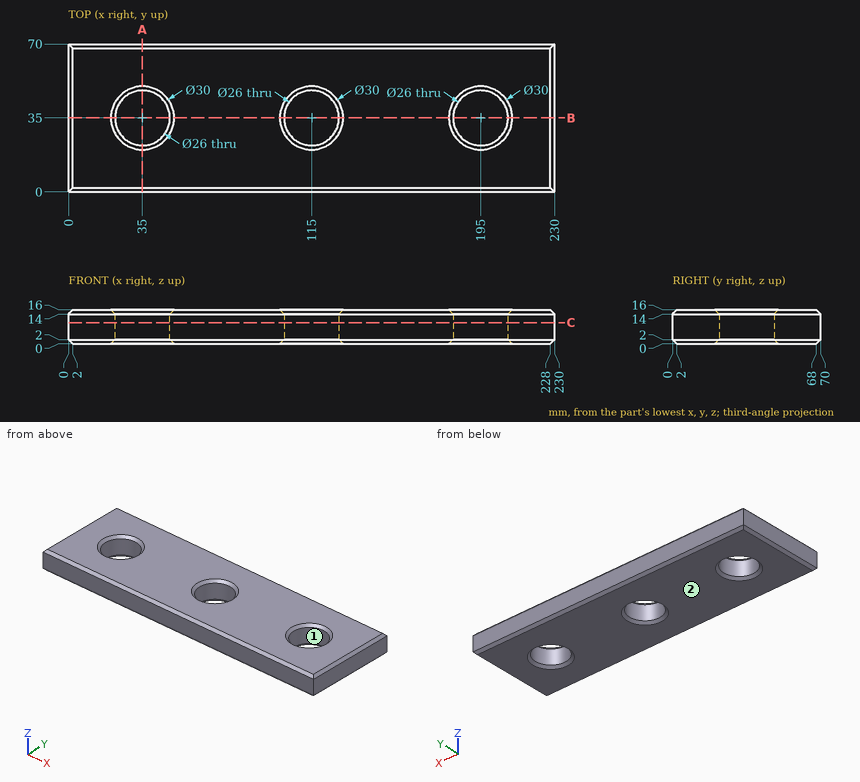
Here's the drawing with two shaded views (mm, measured from the low corner). I have some questions. Round coordinates to 2 decimals unless told otherwise and drop trailing zeros. Order: outer loops, then holes, each group sorted by start corner. A loop starts at its lowest first (then second) coordinate and runs counter-clockwise, first axis right, second up. Notation, with made-up numbers: (82.5, 10) -> (125.5, 10) arc R13 cw to (125.5, 29) -> close; hole circle Ø6 at (-13, 35.5). An arc over 180 degrees is marked (long way). Use a Markdown table: item, result. Add a question column.
(1) Suppose I cut it at C-C, the plane z = 10. Please give me the cut outline in (x, y), and give its area (3 significant figures).
(2) For pin 1 Ø12 at (x, y) = (34, 42.5) entering from -Z; pin 2 Ø10 at (x, y) = (197, 26.5) entering from -Z, each with a flat end and sliding along its axis, tell me the tip position at first contact or that it passes through.
(3) If we mould it in two halves opening along X, with no side actions, what happens to the marked faces 1 and 2? For each: released by +X, released by -X, zero draft, split by the parting line, or undercut.
(4) Suppose I cut it at B-B, the plane y = 35. Count the separate pieces of the cut face and the enclosed holes in it, and give its area (3 significant figures).
(5) I need wall thicknesses on line 1 along X through (y, z) = (34, 6); line 2 along Y through (x, z) = (195, 9); line 3 along X through (y, z) = (41, 6). Which ranges of each line are inside material? Lowest first, please.
(6) Suppose I cut it at A-A, the plane x = 35. Please give me the cut outline in (y, z), and give its area (3 significant figures).
Verdict:
| question | item | result |
|---|---|---|
| 1 | outline | (0, 0) -> (230, 0) -> (230, 70) -> (0, 70) -> close; hole circle Ø26 at (35, 35); hole circle Ø26 at (115, 35); hole circle Ø26 at (195, 35) |
| 1 | area | 14,500 mm2 |
| 2 | pin 1 | z = 1.43 |
| 2 | pin 2 | z = 1.27 |
| 3 | face 1 | undercut |
| 3 | face 2 | zero draft |
| 4 | separate pieces | 4 |
| 4 | enclosed holes | 0 |
| 4 | area | 2,400 mm2 |
| 5 | line 1 | 0 to 22.04, 47.96 to 102.04, 127.96 to 182.04, 207.96 to 230 |
| 5 | line 2 | 0 to 22, 48 to 70 |
| 5 | line 3 | 0 to 23.47, 46.53 to 103.47, 126.53 to 183.47, 206.53 to 230 |
| 6 | outline | (0, 2) -> (2, 0) -> (20, 0) -> (22, 2) -> (22, 14) -> (20, 16) -> (2, 16) -> (0, 14) -> close; (48, 2) -> (50, 0) -> (68, 0) -> (70, 2) -> (70, 14) -> (68, 16) -> (50, 16) -> (48, 14) -> close |
| 6 | area | 688 mm2 |
